from build123d import *

# Parameters (mm, degrees)
BOX004_W               = 147
BOX004_H               = 72
BOX004_DEPTH           = 10
BOX005_W               = 5
BOX005_H               = 72
BOX005_DEPTH           = 15
CYLINDER003_W          = 36
CYLINDER003_H          = 5
CYLINDER003_ANGLE      = 180
BOX006_W               = 5
BOX006_H               = 72
BOX006_DEPTH           = 15
CYLINDER004_W          = 36
CYLINDER004_H          = 5
CYLINDER004_ANGLE      = 180
BOX007_W               = 147
BOX007_H               = 6.4
BOX007_DEPTH           = 22
CYLINDER005_R          = 7
CYLINDER005_DEPTH      = 72
CYLINDER006_R          = 7
CYLINDER006_DEPTH      = 72
CYLINDER007_R          = 3.2
CYLINDER007_DEPTH      = 72
CYLINDER008_R          = 3.2
CYLINDER008_DEPTH      = 72
PRISM001_DEPTH         = 11
PRISM002_DEPTH         = 11
PRISM003_DEPTH         = 11
PRISM004_DEPTH         = 11
POCKET001_DEPTH        = 10
LINEARPATTERN001_COUNT = 4
LINEARPATTERN001_PITCH = 14


with BuildPart() as part:
    # Box004 → Box004 (join)
    with BuildSketch(Plane.XY):
        with Locations((73.5, 36)):
            Rectangle(BOX004_W, BOX004_H)
    extrude(amount=BOX004_DEPTH)

    # Box005 → Box005 (join)
    with BuildSketch(Plane.XY.offset(10)):
        with Locations((2.5, 36)):
            Rectangle(BOX005_W, BOX005_H)
    extrude(amount=BOX005_DEPTH)

    # Cylinder003 → Cylinder003 (revolve)
    with BuildSketch(Plane(origin=(0, 36, 25), x_dir=(0, 1, 0), z_dir=(0, 0, -1))):
        with Locations((18, 2.5)):
            Rectangle(CYLINDER003_W, CYLINDER003_H)
    revolve(axis=Axis((0, 36, 25), (1, 0, 0)), revolution_arc=CYLINDER003_ANGLE)

    # Box006 → Box006 (join)
    with BuildSketch(Plane(origin=(142, 0, 10), x_dir=(1, 0, 0), z_dir=(0, 0, 1))):
        with Locations((2.5, 36)):
            Rectangle(BOX006_W, BOX006_H)
    extrude(amount=BOX006_DEPTH)

    # Cylinder004 → Cylinder004 (revolve)
    with BuildSketch(Plane(origin=(142, 36, 25), x_dir=(0, 1, 0), z_dir=(0, 0, -1))):
        with Locations((18, 2.5)):
            Rectangle(CYLINDER004_W, CYLINDER004_H)
    revolve(axis=Axis((142, 36, 25), (1, 0, 0)), revolution_arc=CYLINDER004_ANGLE)

    # Box007 → Box007 (cut)
    with BuildSketch(Plane(origin=(0, 32.8, 39), x_dir=(1, 0, 0), z_dir=(0, 0, 1))):
        with Locations((73.5, 3.2)):
            Rectangle(BOX007_W, BOX007_H)
    extrude(amount=BOX007_DEPTH, mode=Mode.SUBTRACT)

    # Cylinder005 → Cylinder005 (join)
    with BuildSketch(Plane(origin=(35, 72, 10), x_dir=(1, 0, 0), z_dir=(0, -1, 0))):
        Circle(CYLINDER005_R)
    extrude(amount=CYLINDER005_DEPTH)

    # Cylinder006 → Cylinder006 (join)
    with BuildSketch(Plane(origin=(112, 72, 10), x_dir=(1, 0, 0), z_dir=(0, -1, 0))):
        Circle(CYLINDER006_R)
    extrude(amount=CYLINDER006_DEPTH)

    # Cylinder007 → Cylinder007 (cut)
    with BuildSketch(Plane(origin=(35, 72, 10), x_dir=(1, 0, 0), z_dir=(0, -1, 0))):
        Circle(CYLINDER007_R)
    extrude(amount=CYLINDER007_DEPTH, mode=Mode.SUBTRACT)

    # Cylinder008 → Cylinder008 (cut)
    with BuildSketch(Plane(origin=(112, 72, 10), x_dir=(1, 0, 0), z_dir=(0, -1, 0))):
        Circle(CYLINDER008_R)
    extrude(amount=CYLINDER008_DEPTH, mode=Mode.SUBTRACT)

    # Prism001 → Prism001 (join)
    with BuildSketch(Plane(origin=(5, 7, 13), x_dir=(0, 1, 0), z_dir=(1, 0, 0))):
        Polygon((14, 0), (-7, 12.124356), (-7, -12.124356), align=None)
    extrude(amount=PRISM001_DEPTH)

    # Prism002 → Prism002 (join)
    with BuildSketch(Plane(origin=(131, 7, 13), x_dir=(0, 1, 0), z_dir=(1, 0, 0))):
        Polygon((14, 0), (-7, 12.124356), (-7, -12.124356), align=None)
    extrude(amount=PRISM002_DEPTH)

    # Prism003 → Prism003 (join)
    with BuildSketch(Plane(origin=(131, 65, 13), x_dir=(0, -1, 0), z_dir=(1, 0, 0))):
        Polygon((14, 0), (-7, 12.124356), (-7, -12.124356), align=None)
    extrude(amount=PRISM003_DEPTH)

    # Prism004 → Prism004 (join)
    with BuildSketch(Plane(origin=(5, 65, 13), x_dir=(0, -1, 0), z_dir=(1, 0, 0))):
        Polygon((14, 0), (-7, 12.124356), (-7, -12.124356), align=None)
    extrude(amount=PRISM004_DEPTH)

    # Sketch001 → Pocket001 (cut)
    with BuildSketch(Plane.XY):
        with BuildLine():
            ThreePointArc((52, 20), (47, 15), (52, 10))
            Line((52, 10), (95, 10))
            ThreePointArc((95, 10), (100, 15), (95, 20))
            Line((95, 20), (52, 20))
        make_face()
    pocket001 = extrude(amount=POCKET001_DEPTH, mode=Mode.SUBTRACT)

    # LinearPattern001: Pocket001 ×4
    with Locations(*[(0, i * LINEARPATTERN001_PITCH, 0) for i in range(1, LINEARPATTERN001_COUNT)]):
        add(pocket001, mode=Mode.SUBTRACT)


with BuildPart() as part_1:
    # Body003 placement: moved
    add(part.part.moved(Location((-16, -5, -39))))


solid = part_1.part
Geometry: final body of the model. Coordinates: model frame, mm. A direction names the side the tool comes from. Round coordinates to 2 decimals unless told otherwise and drop trailing zeros. Loops run counter-clockwise (first coordinate to the right, second up) from the corner with the lowest first, then second, coordinate; pieces in that order, holes last.
Q1. Pull-direction query (Z, two-part tool) for faces 4 (the flat face through (-5.58, 56.65, -19.85)), 5 (the cylindrical face through (16.64, 31.5, -26.84)), 6 (the flat face through (-14, 34.2, 11)); classes: released by +Z, released by -Z, zero draft, split by the parting line, or undercut.
Q2. Pin query (flat end, axial travel): P1, Ø12, axis at x = 50.5, z = -21, coming from the -Y side; P2, Ø2.5, axis at x = -14, z = 9, coming from the +Y side; P3, Ø4, axis at x = 129.5, z = 6.5, coming from the +Y side; P4, Ø1.5, axis at x = 94, y = 52, coming from the +Z side. Return the tip coordinate at first contact, or that it passes through.
Q3. Section D-D on x = 19. Return loops of the section in (y, z).
Q4. Material intervals for L1, parallel to Z at x = 19, y = 35; L2, parallel to X at y = 44, z = -20; L3, parallel to Z at x = 104, y = 57.5, sorted ascending.
Q5. Access query for faces 1 (the flat face through (57, 32, -29)), 2 (the flat face through (-5.577, 5.647, -20.023)), 3 (the flat face through (58, 29, -34)). Directions: +Z, -Z, +X, -X, +Y, -Y. A direction counts if a zero-diameter tool reaches every point of the face in a straight line with its end or side. Return the directions, or none.
Q6. Section C-C on y = 38. Return loops of the section in (x, z).
Q7. Section A-A on x = 52. Return loops of the section in (y, z).
Q8. Section B-B on z = 11.5. Return loops of the section in (x, y), plus the area to 3 significant figures.
Evaluation:
1. face 4: released by +Z
1. face 5: undercut
1. face 6: zero draft
2. P1: passes through
2. P2: stops at y = 59.69
2. P3: stops at y = 61.88
2. P4: stops at z = -22.11
3. outline: (-5, -39) - (67, -39) - (67, -32.2) - (-5, -32.2) - close; (-5, -25.8) - (67, -25.8) - (67, -22) - (-5, -22) - close
4. L1: z = -39 to -32.2, -25.8 to -22
4. L2: x = -16 to -11, 126 to 131
4. L3: z = -39 to -29
5. face 1: +Z, +Y, -Y
5. face 2: +Z
5. face 3: +Z, -Z
6. outline: (-16, -39) - (31, -39) - (31, -29) - (26, -29) arc R7 ccw to (12, -29) - (-11, -29) - (-11, 21.31) - (-16, 21.31) - close; (84, -39) - (131, -39) - (131, 21.31) - (126, 21.31) - (126, -29) - (103, -29) arc R7 ccw to (89, -29) - (84, -29) - close; hole circle Ø6.4 at (19, -29); hole circle Ø6.4 at (96, -29)
7. outline: (-5, -39) - (5, -39) - (5, -29) - (-5, -29) - close; (15, -39) - (19, -39) - (19, -29) - (15, -29) - close; (29, -39) - (33, -39) - (33, -29) - (29, -29) - close; (43, -39) - (47, -39) - (47, -29) - (43, -29) - close; (57, -39) - (67, -39) - (67, -29) - (57, -29) - close
8. outline: (-16, 5.59) - (-11, 5.59) - (-11, 27.8) - (-16, 27.8) - close; (-16, 34.2) - (-11, 34.2) - (-11, 56.41) - (-16, 56.41) - close; (126, 5.59) - (131, 5.59) - (131, 27.8) - (126, 27.8) - close; (126, 34.2) - (131, 34.2) - (131, 56.41) - (126, 56.41) - close
8. area: 444 mm2
